Geometry check sheet. Reference: the model listing, model coordinates, mm. Give positions to 0.01 mm unless a question says otherwise; leave off trailing zeros. Loops run counter-clockwise (first coordinate to the right, second up) from the corner with the lowest first, then second, coordinate; pieces in that order, holes last. Notation, with made-up numbers: (79, 40) -> (134, 40) arc R23 ccw to (134, 68) -> close; hole circle Ø4 at (28, 24.25). An arc over 180 degrees is marked (long way). Answer as a JSON object with one key per item and string values.
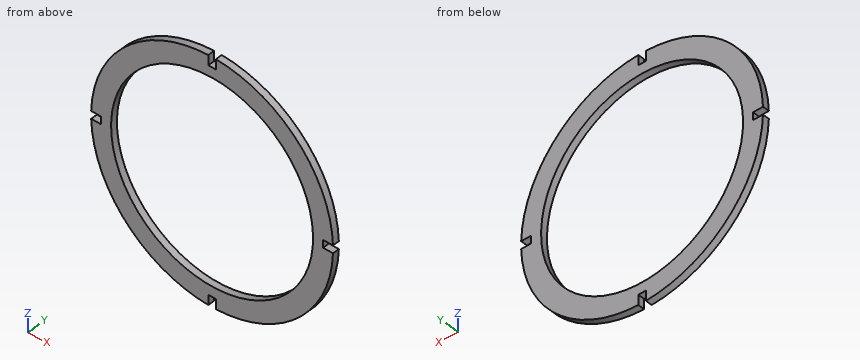
from build123d import *

# Parameters (mm, degrees)
SKETCH1_R           = 45.5
BOSS_EXTRUDE1_DEPTH = 1.5


with BuildPart() as part:
    # Sketch1 → Boss-Extrude1 (new, symmetric)
    with BuildSketch(Plane(origin=(0, 0, 0), x_dir=(1, 0, 0), z_dir=(0, 1, 0))):
        with BuildLine():
            Line((-1.7, 54.473479786), (-1.7, 50))
            Line((-1.7, 50), (1.7, 50))
            Line((1.7, 50), (1.7, 54.473479786))
            ThreePointArc((1.7, 54.473479786), (38.537319575, 38.537319575), (54.473479786, 1.7))
            Line((54.473479786, 1.7), (50, 1.7))
            Line((50, 1.7), (50, -1.7))
            Line((50, -1.7), (54.473479786, -1.7))
            ThreePointArc((54.473479786, -1.7), (38.537319575, -38.537319575), (1.7, -54.473479786))
            Line((1.7, -54.473479786), (1.7, -50))
            Line((1.7, -50), (-1.7, -50))
            Line((-1.7, -50), (-1.7, -54.473479786))
            ThreePointArc((-1.7, -54.473479786), (-38.537319575, -38.537319575), (-54.473479786, -1.7))
            Line((-54.473479786, -1.7), (-50, -1.7))
            Line((-50, -1.7), (-50, 1.7))
            Line((-50, 1.7), (-54.473479786, 1.7))
            ThreePointArc((-54.473479786, 1.7), (-38.537319575, 38.537319575), (-1.7, 54.473479786))
        make_face()
        with Locations(Location((0, 0, 0), (0, 0, 270))):
            Circle(SKETCH1_R, mode=Mode.SUBTRACT)
    extrude(amount=BOSS_EXTRUDE1_DEPTH, both=True)


solid = part.part
1) Section check B-B on x = 0. Record the cut outline in (y, z), plus the area to 3 significant figures.
Geometry check:
{"outline": "(-1.5, -50) -> (1.5, -50) -> (1.5, -45.5) -> (-1.5, -45.5) -> close; (-1.5, 45.5) -> (1.5, 45.5) -> (1.5, 50) -> (-1.5, 50) -> close", "area": "27.0 mm2"}
2) Material ranges on line 1 along X through (y, z) = (-0.15, 0); line 2 along X through (y, z) = (-1, -35); line 3 along Z through (x, y) = (-40, -1.3), recorded low to high. Write a range as from..to.
Geometry check:
{"line 1": "x = -50..-45.5, 45.5..50", "line 2": "x = -41.78..-29.07, 29.07..41.78", "line 3": "z = -37.02..-21.69, 21.69..37.02"}
3) Depth check by flat-ended pin: P1, Ø0.9, axis at y = -0.5, z = 0.5, coming from the -X side; P2, Ø0.9, axis at y = 0.5, z = 0, coming from the +X side; P3, Ø1, axis at x = 11, y = 0, coming from the +Z side. Enter the tip coordinate at first touch or a pass-through.
Geometry check:
{"P1": "stops at x = -50", "P2": "stops at x = 50", "P3": "stops at z = 53.48"}
4) Section check C-C on z = 0. Record the cut outline in (x, y), plus the area to 3 significant figures.
Geometry check:
{"outline": "(-50, -1.5) -> (-45.5, -1.5) -> (-45.5, 1.5) -> (-50, 1.5) -> close; (45.5, -1.5) -> (50, -1.5) -> (50, 1.5) -> (45.5, 1.5) -> close", "area": "27.0 mm2"}
5) Section check A-A on y = -0.6. Record the cut outline in (x, z), plus the area to 3 significant figures.
Geometry check:
{"outline": "(-54.47, -1.7) arc R54.5 ccw to (-1.7, -54.47) -> (-1.7, -50) -> (1.7, -50) -> (1.7, -54.47) arc R54.5 ccw to (54.47, -1.7) -> (50, -1.7) -> (50, 1.7) -> (54.47, 1.7) arc R54.5 ccw to (1.7, 54.47) -> (1.7, 50) -> (-1.7, 50) -> (-1.7, 54.47) arc R54.5 ccw to (-54.47, 1.7) -> (-50, 1.7) -> (-50, -1.7) -> close; hole circle Ø91 at (0, 0)", "area": "2,770 mm2"}
